For this review, take the finished solid that the model builds, in its own axes (mm). Give positions to 0.01 mm unless a question says otherwise; leave off trailing zeros. Order: outer loops, then holes, each group sorted by start corner. A loop starts at its lowest first (then second) coordinate and runs counter-clockwise, first axis right, second up. Notation, with made-up numbers: M 59,-26 L 95,-26 A15 ccw 95,-10 Z; hole C 54,-13 d6. An arc over 180 degrees is marked long. Use CSV: the item, a comma, the result in double quotes. Start each with the question number.
(1) Consider section C-C (y = 0). Write out the cut boundary in (x, z).
(2) Draft analysis for pull direction Y (two halves, no side actions). For faces 1 (the face through (2, -4.2, 29)), 2 (the face through (0, 0, 1)), state which applies: pulls with the +Y half, pulls with the -Y half, needs draft (parallel to the pull), parting line crosses it, or undercut.
(3) Consider section D-D (x = 2.25). Give the number of separate pieces and of enclosed holes in the cut face, and give its area (3 significant figures).
(4) Consider section A-A (y = 8). Write out the cut boundary in (x, z).
(5) Consider section B-B (z = 57.5). Write out the cut boundary in (x, y), and give its area (3 significant figures).
(6) Wall thickness on L1, parallel to Z at x = 0.35, y = -17.5; L2, parallel to Y at x = 1.25, z = 57.5; L3, parallel to Z at x = 0.15, y = 0.5: over which ranges is each line inside the solid? List them lowest first. Write a range as from..to.
```python
from build123d import *

# Parameters (mm, degrees)
SKETCH1_W            = 120
SKETCH1_H            = 42
SKETCH1_R            = 1.5
SKETCH1_W_2          = 10
SKETCH1_H_2          = 3
BOSS_EXTRUDE1_DEPTH  = 3
SKETCH2_W            = 3
SKETCH2_H            = 3
CUT_EXTRUDE1_DEPTH   = 3
LPATTERN1_COUNT      = 6
LPATTERN1_PITCH      = 5.4
LPATTERN1_COUNT_DIR2 = 6
LPATTERN1_PITCH_DIR2 = 5.4


with BuildPart() as part:
    # Sketch1 → Boss-Extrude1 (new body)
    with BuildSketch(Plane(origin=(0, 0, 0), x_dir=(0, 0, -1), z_dir=(1, 0, 0))):
        Rectangle(SKETCH1_W, SKETCH1_H)
        with Locations((-57.5, 0)):
            Circle(SKETCH1_R, mode=Mode.SUBTRACT)
        with Locations((57.5, 0)):
            Circle(SKETCH1_R, mode=Mode.SUBTRACT)
        with Locations((25, 18.5)):
            Rectangle(SKETCH1_W_2, SKETCH1_H_2, mode=Mode.SUBTRACT)
        with Locations((-25, 18.5)):
            Rectangle(SKETCH1_W_2, SKETCH1_H_2, mode=Mode.SUBTRACT)
        with Locations((-25, -18.5)):
            Rectangle(SKETCH1_W_2, SKETCH1_H_2, mode=Mode.SUBTRACT)
        with Locations((25, -18.5)):
            Rectangle(SKETCH1_W_2, SKETCH1_H_2, mode=Mode.SUBTRACT)
    extrude(amount=BOSS_EXTRUDE1_DEPTH)

    # Sketch2 → Cut-Extrude1 (cut)
    with BuildSketch(Plane(origin=(3, 0, 0), x_dir=(0, 0, -1), z_dir=(1, 0, 0))):
        with Locations((-12.5, 13.5)):
            Rectangle(SKETCH2_W, SKETCH2_H)
    cut_extrude1 = extrude(amount=-CUT_EXTRUDE1_DEPTH, mode=Mode.SUBTRACT)

    # LPattern1: Cut-Extrude1 6 × 6
    with Locations(*[(0, -j * LPATTERN1_PITCH_DIR2, i * LPATTERN1_PITCH) for i in range(LPATTERN1_COUNT) for j in range(LPATTERN1_COUNT_DIR2) if (i, j) != (0, 0)]):
        add(cut_extrude1, mode=Mode.SUBTRACT)


solid = part.part
```
Check result:
1,outline,"M 0,-60 L 3,-60 L 3,-59 L 0,-59 Z; M 0,-56 L 3,-56 L 3,56 L 0,56 Z; M 0,59 L 3,59 L 3,60 L 0,60 Z"
2,face 1,"undercut"
2,face 2,"needs draft"
3,separate pieces,"1"
3,enclosed holes,"42"
3,area,"4,580 mm^2"
4,outline,"M 0,-60 L 3,-60 L 3,11 L 0,11 Z; M 0,14 L 3,14 L 3,16.4 L 0,16.4 Z; M 0,19.4 L 3,19.4 L 3,21.8 L 0,21.8 Z; M 0,24.8 L 3,24.8 L 3,27.2 L 0,27.2 Z; M 0,30.2 L 3,30.2 L 3,32.6 L 0,32.6 Z; M 0,35.6 L 3,35.6 L 3,38 L 0,38 Z; M 0,41 L 3,41 L 3,60 L 0,60 Z"
5,outline,"M 0,-21 L 3,-21 L 3,-1.5 L 0,-1.5 Z; M 0,1.5 L 3,1.5 L 3,21 L 0,21 Z"
5,area,"117 mm^2"
6,L1,"z = -60..-30, -20..20, 30..60"
6,L2,"y = -21..-1.5, 1.5..21"
6,L3,"z = -60..-58.91, -56.09..56.09, 58.91..60"
